Geometry: see drawing. Coordinates: mm, zero at the bounding-box minimum. A direction names the side the tool comes from. Coordinates: 2 decimals unless noted, no trailing zeros. Loops run counter-clockwise (first coordinate to the right, second up) from the corner with the lowest first, then second, coordinate; pieces in that order, holes last. Notation, with made-up numbers: (69, -19.5) - (80, -19.5) arc R27 cw to (80, 8.5) - close; hole circle Ø11 at (34.25, 9.5). An arc over 180 degrees is marked (long way). Write each question's results on one line, items separated by ' | '. Start each with the question number.
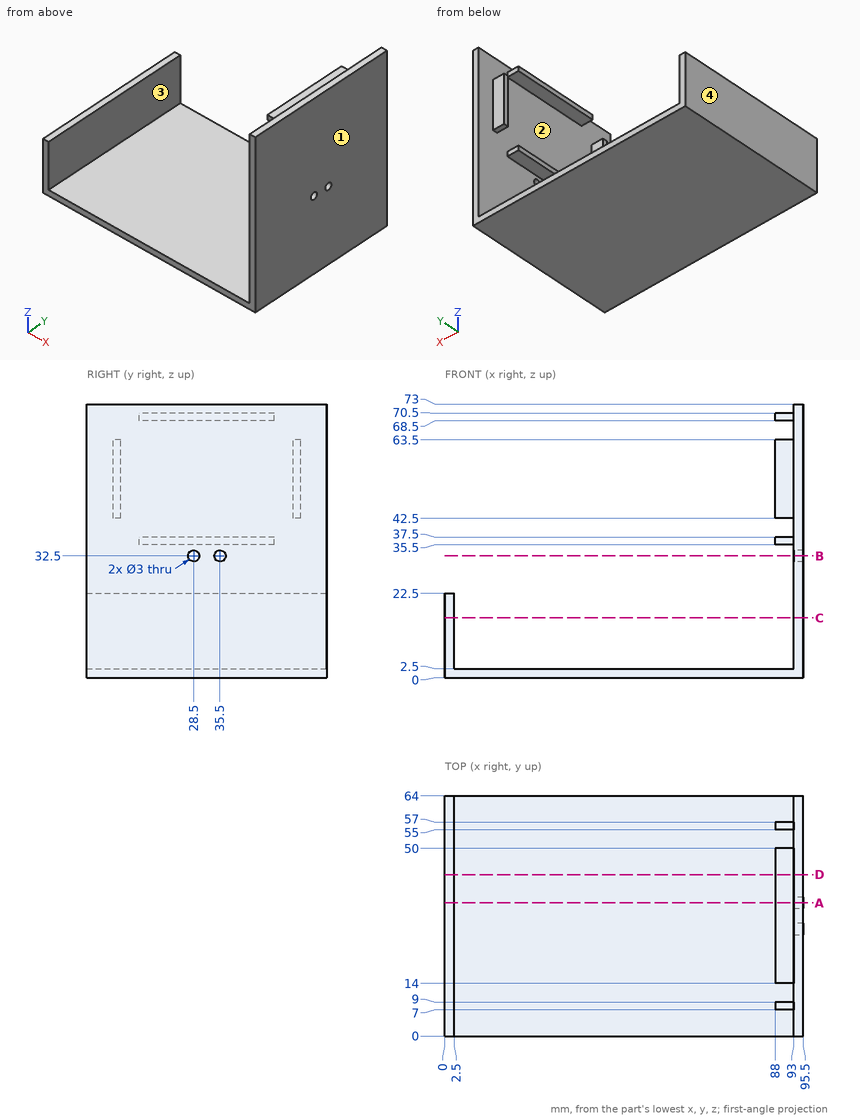
1) Access query for the marked faces 3 and 4. Directions: +Z, -Z, +X, -X, +Y, -Y. A direction counts if a zero-diameter tool reaches every point of the face in a straight line with its end or side. Return the directions, or none.
2) Section query C-C on z = 16. Output: boundary loops of the cut face in (x, y), and give its area (3 significant figures).
3) Material intervals for line 1 (Z direction, x = 94.45, y = 35.5); line 2 (Y direction, x = 88.5, z = 55); line 3 (Y direction, x = 94, z = 32), sorted ascending. Write a range as [from, to].
4) Pin query (flat end, axial travel): pin 1 Ø1 at (x, y) = (40.5, 31) entering from +Z; pin 2 Ø1.6 at (y, z) = (56.5, 54.5) entering from -X; pin 3 Ø1 at (x, y) = (89.5, 7.5) entering from +Z. Return the tip coordinate at first contact, or that it passes through.
5) Section query A-A on y = 35.5. Output: boundary loops of the cut face in (x, z).
6) Pull-direction query (Y, two-part tool) for the marked faces 1 and 2; classes: released by +Y, released by -Y, zero draft, split by the parting line, or undercut.
7) Section query B-B on z = 32.5. Output: boundary loops of the cut face in (x, y).
8) Section query D-D on y = 43. Output: boundary loops of the cut face in (x, z).
Returned:
1) face 3: +Z, +Y, -Y | face 4: +Z, -Z, -X, +Y, -Y
2) outline: (0, 0) - (2.5, 0) - (2.5, 64) - (0, 64) - close; (93, 0) - (95.5, 0) - (95.5, 64) - (93, 64) - close | area: 320 mm²
3) line 1: z = [0, 31], [34, 73] | line 2: y = [7, 9], [55, 57] | line 3: y = [0, 27.09], [29.91, 34.09], [36.91, 64]
4) pin 1: stops at z = 2.5 | pin 2: stops at x = 88 | pin 3: stops at z = 63.5
5) outline: (0, 0) - (95.5, 0) - (95.5, 31) - (93, 31) - (93, 2.5) - (2.5, 2.5) - (2.5, 22.5) - (0, 22.5) - close; (88, 35.5) - (93, 35.5) - (93, 34) - (95.5, 34) - (95.5, 73) - (93, 73) - (93, 70.5) - (88, 70.5) - (88, 68.5) - (93, 68.5) - (93, 37.5) - (88, 37.5) - close
6) face 1: zero draft | face 2: undercut
7) outline: (93, 0) - (95.5, 0) - (95.5, 27) - (93, 27) - close; (93, 30) - (95.5, 30) - (95.5, 34) - (93, 34) - close; (93, 37) - (95.5, 37) - (95.5, 64) - (93, 64) - close
8) outline: (0, 0) - (95.5, 0) - (95.5, 73) - (93, 73) - (93, 70.5) - (88, 70.5) - (88, 68.5) - (93, 68.5) - (93, 37.5) - (88, 37.5) - (88, 35.5) - (93, 35.5) - (93, 2.5) - (2.5, 2.5) - (2.5, 22.5) - (0, 22.5) - close
